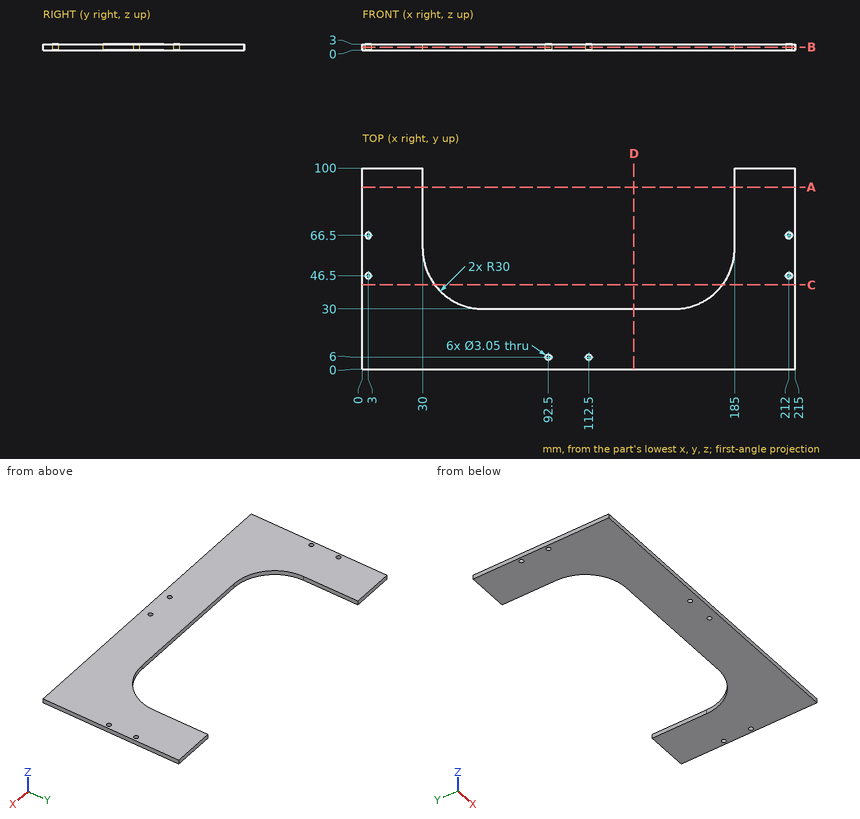
Job drawing, mm, ordinate dimensions from the low corner. One solid piece. Round coordinates to 2 decimals unless told otherwise and drop trailing zeros. Loops run counter-clockwise (first coordinate to the right, second up) from the corner with the lowest first, then second, coordinate; pieces in that order, holes last. Notation, with made-up numbers: (75.5, 88.25) -> (126.5, 88.25) arc R20 ccw to (126.5, 117.25) -> close; hole circle Ø7 at (15, 14.25). An arc over 180 degrees is marked (long way). One line per item, written item: value. Start each with the question number.
Q1. Cut at A-A on y = 90.5. List the corners of the cut face in (x, z).
Q2. Cut at D-D on x = 135. List the corners of the cut face in (y, z), plus the area to 3 significant figures.
Q3. Cut at B-B on z = 1.4. List the corners of the cut face in (x, y) (3 decimals), plus the area to 3 significant figures.
Q4. Probe line 1 along Y through (x, z) = (212, 2.2) (3 decimals); line 2 along X through (y, z) = (61, 0.85); line 3 along Y through (x, z) = (140, 0.3). List the from-to ranges inside material, lowest first.
Q5. Cut at C-C on y = 42. List the corners of the cut face in (x, z), plus the area to 3 significant figures.
Q6. Drop a flat-ended pin along its axis: pin 1 Ø1.5 at (x, z) = (129.5, 1.5) entering from +Y. Give the stop position or say it passes through.
Computed:
1. outline: (0, 0) -> (30, 0) -> (30, 3) -> (0, 3) -> close; (185, 0) -> (215, 0) -> (215, 3) -> (185, 3) -> close
2. outline: (0, 0) -> (30, 0) -> (30, 3) -> (0, 3) -> close
2. area: 90.0 mm²
3. outline: (0, 0) -> (215, 0) -> (215, 100) -> (185, 100) -> (185, 60) arc R30 cw to (155, 30) -> (60, 30) arc R30 cw to (30, 60) -> (30, 100) -> (0, 100) -> close; hole circle Ø3.05 at (3, 46.5); hole circle Ø3.05 at (3, 66.5); hole circle Ø3.05 at (92.5, 6); hole circle Ø3.05 at (112.5, 6); hole circle Ø3.05 at (212, 46.5); hole circle Ø3.05 at (212, 66.5)
3. area: 11,000 mm²
4. line 1: 0 to 44.975, 48.025 to 64.975, 68.025 to 100
4. line 2: 0 to 30, 185 to 215
4. line 3: 0 to 30
5. outline: (0, 0) -> (36, 0) -> (36, 3) -> (0, 3) -> close; (179, 0) -> (215, 0) -> (215, 3) -> (179, 3) -> close
5. area: 216 mm²
6. pin 1: y = 30
